```python
from build123d import *

# Parameters (mm, degrees)
PAD_DEPTH    = 20
SKETCH001_W  = 5
SKETCH001_H  = 2
POCKET_DEPTH = 20.001
FILLET_R     = 1.9999


with BuildPart() as part:
    # Sketch → Pad (new body)
    with BuildSketch(Plane.XY):
        with BuildLine():
            Line((15, 0), (15, -2))
            ThreePointArc((12, -5), (14.12132, -4.12132), (15, -2))
            Line((12, -5), (-12, -5))
            ThreePointArc((-15, -2), (-14.12132, -4.12132), (-12, -5))
            Line((-15, -2), (-15, 0))
            ThreePointArc((-6.917175, 13.309872), (-12.82103, 7.785961), (-15, 0))
            ThreePointArc((-6.917175, 13.309872), (-5.151623, 14.961802), (-4.5, 17.290199))
            Line((-4.5, 17.290199), (-4.5, 19.290199))
            Line((-4.5, 19.290199), (4.5, 19.290199))
            Line((4.5, 19.290199), (4.5, 17.290199))
            ThreePointArc((4.5, 17.290199), (5.151623, 14.961802), (6.917175, 13.309872))
            ThreePointArc((15, 0), (12.82103, 7.785961), (6.917175, 13.309872))
        make_face()
        with BuildLine():
            Line((-10, -3), (10, -3))
            ThreePointArc((10, -3), (12.12132, -2.12132), (13, 0))
            ThreePointArc((13, 0), (11.111559, 6.747833), (5.994885, 11.535222))
            ThreePointArc((2.5, 17.290199), (3.442152, 13.923674), (5.994885, 11.535222))
            Line((-2.5, 17.290199), (2.5, 17.290199))
            ThreePointArc((-5.994885, 11.535222), (-3.442152, 13.923674), (-2.5, 17.290199))
            ThreePointArc((-5.994885, 11.535222), (-11.111559, 6.747833), (-13, 0))
            ThreePointArc((-13, 0), (-12.12132, -2.12132), (-10, -3))
        make_face(mode=Mode.SUBTRACT)
    extrude(amount=PAD_DEPTH)

    # Sketch001 (on Face22 of Pad) → Pocket (cut, through all)
    with BuildSketch(Plane.XY.offset(20)):
        with Locations((0, 18.290199)):
            Rectangle(SKETCH001_W, SKETCH001_H)
    extrude(amount=-POCKET_DEPTH, mode=Mode.SUBTRACT)

    # Fillet
    fillet_edges = [part.edges().sort_by_distance(p)[0] for p in [
        (-2.5, 19.290199, 10),
        (2.5, 19.290199, 10),
    ]]
    fillet(fillet_edges, radius=FILLET_R)


solid = part.part
```
Here's how the part is built. I have some questions about the finished solid (model axes, mm). A direction names the side the tool comes from. Give positions to 0.01 mm unless a question says otherwise; leave off trailing zeros. Loops run counter-clockwise (first coordinate to the right, second up) from the corner with the lowest first, then second, coordinate; pieces in that order, holes last. Notation, with made-up numbers: M 44.5,-25.75 L 62.5,-25.75 A30 ccw 62.5,4.25 Z; hole C 34.25,37.25 d6. An arc over 180 degrees is marked long. Use one line per item in the form item = value. Start each with the question number.
Q1. Will these pins go through, and if not, where does the flat tip stop? pin 1 Ø1 at (y, z) = (18, 14.5) entering from -X; pin 2 Ø4 at (y, z) = (7.5, 13.5) entering from +X; pin 3 Ø1 at (x, y) = (-7.5, 14) entering from +Z; pin 4 Ø2 at (y, z) = (5.5, 12) entering from -X.
Q2. If we section it at D-D (x = 2): Write out the boundary of the cut face in (y, z).
Q3. Thinking about a two-plate mould opening in X: for faces 4 (the cylindrical face through (12.1, -2.14, 9.86)), 5 (the flat face through (-15, -1, 10)), 6 (the cylindrical face through (-3.47, 13.88, 9.86)), 7 (the cylindrical face through (5.134, 14.991, 9.86)), which applies, +X half, -X half, draft (parallel to the pull), parting line (faces both ways), or undercut?
Q4. If we section it at A-A (y = 15.25): Write out the boundary of the cut face in (x, z).
Q5. Which directions (+Z, -Z, +X, -X, +Y, -Y) give clear straight access to the entire face, cutting with the end or side of a thin tool? Please do faces 1 (the cylindrical face through (-3.07, 18.69, 9.86)), 2 (the cylindrical face through (3.417, 13.966, 9.86)), 3 (the flat face through (-4.5, 18, 10)).
Q6. I need wall thicknesses on line 1 along X through (y, z) = (12.75, 5); line 2 along X through (y, z) = (14.75, 8.75); line 3 along Y through (x, z) = (-7.5, 9). Which ranges of each line are inside material? Lowest first, please.
Q7. If we section it at B-B (x = -6.5): Write out the boundary of the cut face in (y, z).
Taken from the geometry:
q1.pin_1 = -4.5
q1.pin_2 = 13.96
q1.pin_3 = through
q1.pin_4 = -14.31
q2.outline = M -5,0 L -3,0 L -3,20 L -5,20 Z
q3.face_4 = undercut
q3.face_5 = -X half
q3.face_6 = undercut
q3.face_7 = +X half
q4.outline = M -4.99,0 L -2.83,0 L -2.83,20 L -4.99,20 Z; M 2.83,0 L 4.99,0 L 4.99,20 L 2.83,20 Z
q5.face_1 = +Z, -Z, +Y
q5.face_2 = +Z, -Z
q5.face_3 = +Z, -Z, -X, +Y
q6.line_1 = -7.9 to -4.35, 4.35 to 7.9
q6.line_2 = -5.29 to -3.02, 3.02 to 5.29
q6.line_3 = -5 to -3, 10.62 to 12.99
q7.outline = M -5,0 L -3,0 L -3,20 L -5,20 Z; M 11.26,0 L 13.56,0 L 13.56,20 L 11.26,20 Z
